Check sheet for the modelled part. Datum: model origin and axes. Units: mm. Face numbers are marked on the shaded views. A direction names the side the tool comes from. Give positions to 0.01 mm unless a question says otherwise; leave off trailing zeros. Order: outer loops, then holes, each group sorted by start corner. A loop starts at its lowest first (then second) coordinate and runs counter-clockwise, first axis right, second up.
Item 1: Sectioned sample at A-A on x = 0. Record the boundary of the cut face in (y, z), and give its area (3 significant figures).
Item 2: Access from +Z, -Z, +X, -X, +Y, -Y to the whole of each face (thin tool, end or side, straight path). Record for the marked faces 4 and 5.
Item 3: Sectioned sample at C-C on z = 3.25. Record the boundary of the cut face in (x, y).
Item 4: Material ranges on line 1 along Y through (x, z) = (0, 13); line 2 along X through (y, z) = (-0.75, 1.75); line 3 along Y through (x, z) = (-2, 13), recorded low to high.
Item 5: Release check for a two-part mould opening along X. For the marked faces 1, 2 and 3 record: released by +X, released by -X, zero draft, split by the parting line, or undercut.
Item 6: Sectioned sample at D-D on z = 22.5. Record the boundary of the cut face in (x, y), and give its area (3 significant figures).
Item 7: Gauge pin test, flat ends, axial feed: P1, Ø1, axis at x = -1.5, z = 10, coming from the +Y side; P2, Ø2, axis at x = -2.5, z = 8, coming from the +Y side; P3, Ø1.5, axis at x = -0.5, y = 0.5, coming from the -Z side. Record the tip position at first contact, or that the pin passes through.
Item 8: Sectioned sample at B-B on y = 0. Record the boundary of the cut face in (x, z).
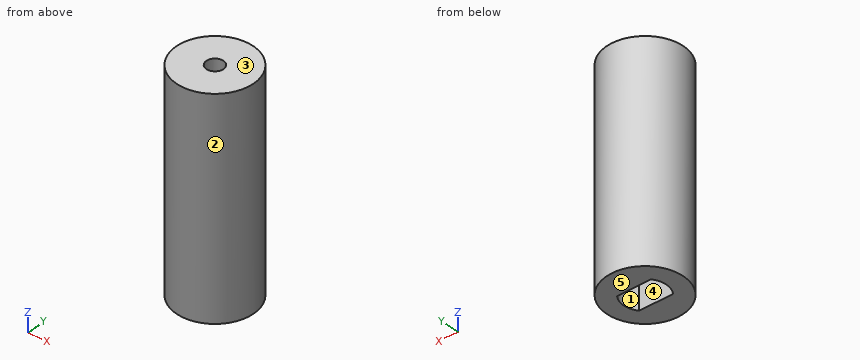
Solid Edge part; units mm, degrees
sketch "Sketch1" plane through (0, 0, 0) normal (0, 0, 1) x (1, 0, 0)
  circle A0 centre (0, 0) radius 4.5
extrude "Protrusion1" add sketch "Sketch1" along normal blind 25
sketch "Sketch2" plane through (0, 0, 0) normal (0, 0, -1) x (1, 0, 0)
  line L0 (2, -1.5) -> (-2, -1.5)
  line L1 (-2, 1.5) -> (2, 1.5)
  arc A0 (2, 1.5) -> (2, -1.5) centre (0, 0) cw
  arc A1 (-2, -1.5) -> (-2, 1.5) centre (0, 0) cw
extrude "ExtrudedCutout_1" cut sketch "Sketch2" against normal blind 6 and the other way blind 2.1211
sketch "Sketch3" plane through (0, 0, 25) normal (0, 0, 1) x (1, 0, 0)
  circle A0 centre (0, 0) radius 1
extrude "ExtrudedCutout_2" cut sketch "Sketch3" against normal blind 37.6627 and the other way blind 30.582
Report:
1. outline: (-4.5, 0) - (-1.5, 0) - (-1.5, 6) - (-1, 6) - (-1, 25) - (-4.5, 25) - close; (1, 6) - (1.5, 6) - (1.5, 0) - (4.5, 0) - (4.5, 25) - (1, 25) - close
1. area: 169 mm2
2. face 4: -Z
2. face 5: -Z, +X, -X, +Y, -Y
3. outline: circle Ø9 at (0, 0); hole (-2, -1.5) - (2, -1.5) arc R2.5 ccw to (2, 1.5) - (-2, 1.5) arc R2.5 ccw to start
4. line 1: y = -4.5 to -1, 1 to 4.5
4. line 2: x = -4.44 to -2.38, 2.38 to 4.44
4. line 3: y = -4.03 to 4.03
5. face 1: undercut
5. face 2: split by the parting line
5. face 3: zero draft
6. outline: circle Ø9 at (0, 0); hole circle Ø2 at (0, 0)
6. area: 60.5 mm2
7. P1: stops at y = 4.39
7. P2: stops at y = 4.24
7. P3: stops at z = 6
8. outline: (-4.5, 0) - (-2.5, 0) - (-2.5, 6) - (-1, 6) - (-1, 25) - (-4.5, 25) - close; (1, 6) - (2.5, 6) - (2.5, 0) - (4.5, 0) - (4.5, 25) - (1, 25) - close
